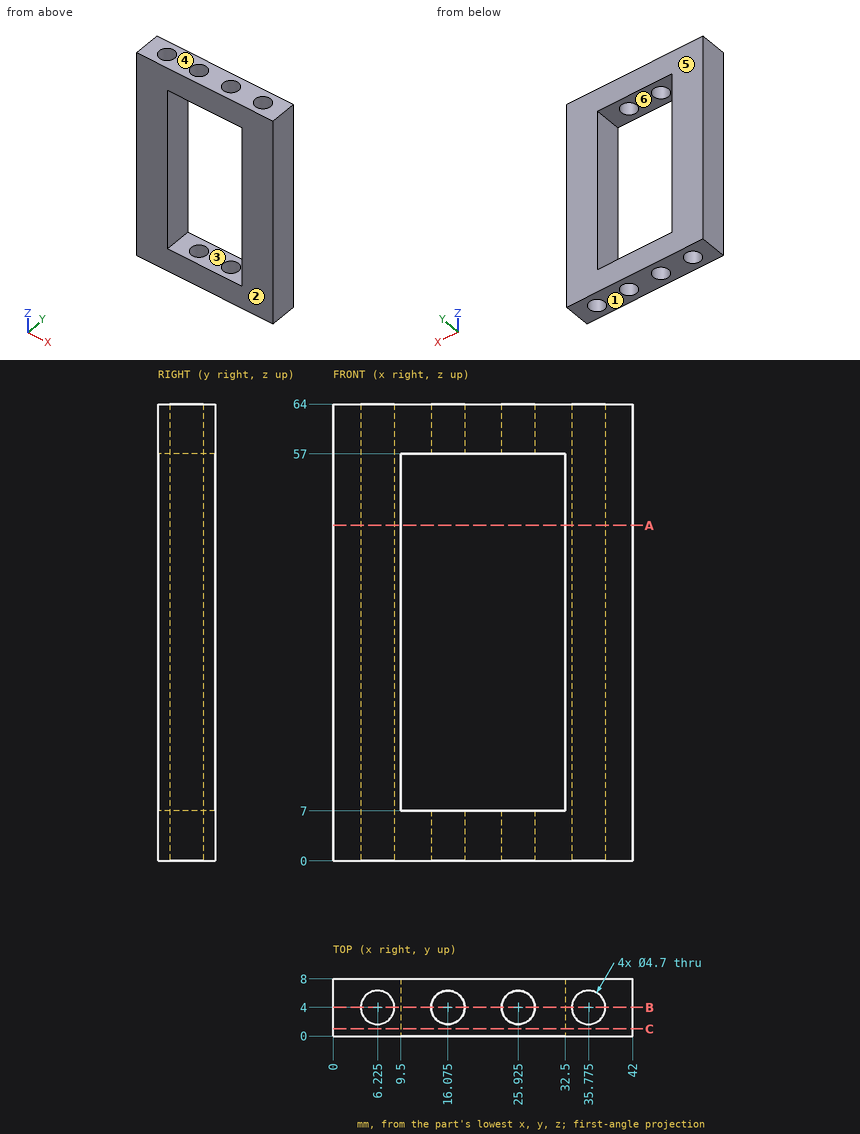
Geometry check sheet. Reference: drawing and pictorial views, mm from the part's lowest x, y, z. A direction names the side the tool comes from. Give positions to 0.01 mm unless a question says otherwise; leave off trailing zeros. Loops run counter-clockwise (first coordinate to the right, second up) from the corner with the lowest first, then second, coordinate; pieces in that order, holes last. Notation, with made-up numbers: M -36.75,8.5 L -22.75,8.5 A12 ccw -22.75,21.5 Z; hole C 72,49 d7. An arc over 180 degrees is marked long. Use a Markdown table: item, result. Add a question column.
Q1. Sectioned sample at A-A, the plane z = 47. Record the cut outline in (x, y) (3 decimals).
Q2. Mould release check, pull along Z, two halves, no side actions. Record for the marked faces 1, 2, 3 and 4: pulls with the +Z half, pulls with the -Z half, needs draft (parallel to the pull), parting line crosses it, or undercut.
Q3. Tool access check on the marked faces 5 and 6. Record the directions out of +Z, -Z, +X, -X, +Y, -Y that give a thin tool (end or side, any length) a straight path to the whole face; none if there is none.
Q4. Go/stop test with a flat-tipped pin: pin 1 (6 mm diameter, centred on x = 10.5, z = 41, fed in from -Y). Record where the tip stops, or that it passes through.
Q5. Scan lines: line 1 along X through (y, z) = (6.75, 32); line 2 along Y through (x, z) = (36, 29); line 3 along Z through (x, y) = (12, 2.5). Record each from-to range of solid material in increasing order. Write a range as [from, to].
Q6. Sectioned sample at C-C, the plane y = 1. Record the cut outline in (x, z).
Q7. Sectioned sample at B-B, the plane y = 4. Give the number of separate pieces and of enclosed holes in the cut face, then the cut area to 3 significant figures.
Verdict:
| question | item | result |
|---|---|---|
| 1 | outline | M 0,0 L 9.5,0 L 9.5,8 L 0,8 Z; M 32.5,0 L 42,0 L 42,8 L 32.5,8 Z; hole C 6.225,4 d4.7; hole C 35.775,4 d4.7 |
| 2 | face 1 | pulls with the -Z half |
| 2 | face 2 | needs draft |
| 2 | face 3 | undercut |
| 2 | face 4 | pulls with the +Z half |
| 3 | face 5 | +Z, -Z, +X, -X, +Y |
| 3 | face 6 | +Y, -Y |
| 4 | pin 1 | y = 0 |
| 5 | line 1 | [0, 9.5], [32.5, 42] |
| 5 | line 2 | [0, 1.66], [6.34, 8] |
| 5 | line 3 | [0, 7], [57, 64] |
| 6 | outline | M 0,0 L 42,0 L 42,64 L 0,64 Z; hole M 9.5,7 L 32.5,7 L 32.5,57 L 9.5,57 Z |
| 7 | separate pieces | 6 |
| 7 | enclosed holes | 0 |
| 7 | area | 805 mm^2 |
